Build history of the part. All positions in model axes, mm. Face numbers are marked on the shaded views. A direction names the side the tool comes from. Coordinates: 2 decimals unless noted, no trailing zeros. Order: outer loops, then holes, each group sorted by start corner. A loop starts at its lowest first (then second) coordinate and runs counter-clockwise, first axis right, second up. Notation, with made-up numbers: (-25.75, 57.5) - (-7.75, 57.5) arc R17 ccw to (-7.75, 79.5) - close; hole circle Ø5 at (-19, -26.5). An arc over 180 degrees is marked (long way). One line per item, written item: value.
from build123d import *

# Parameters (mm, degrees)
F0_W           = 15
F0_H           = 2
F1_DEPTH       = 54
F2_W           = 8.5
F2_H           = 15
F3_DEPTH       = 12.5
F5_D           = 3
F5_DEPTH       = 18
F5_CBORE_D     = 6.5
F5_CBORE_DEPTH = 1.5
F5_TIP         = 0.9012909285
F7_D           = 3
F7_DEPTH       = 18
F7_CBORE_D     = 6.5
F7_CBORE_DEPTH = 1.5
F7_TIP         = 0.9012909285
F8_R           = 4
F9_DEPTH       = 10


with BuildPart() as f1:
    # F0 (on Top) → F1 (new body)
    with BuildSketch(Plane.XY):
        with BuildLine():
            Line((0, 5), (0, 0))
            Line((0, 0), (40, 0))
            Line((40, 0), (40, 25))
            Line((40, 25), (0, 25))
            Line((0, 25), (0, 20))
            ThreePointArc((0, 20), (5.3033008589, 17.8033008589), (7.5, 12.5))
            ThreePointArc((7.5, 12.5), (5.3033008589, 7.1966991411), (0, 5))
        make_face()
        Polygon((12.5, 13.5), (12.5, 22), (27.5, 22), (27.5, 13.5), (27.5, 11.5), (27.5, 3), (12.5, 3), (12.5, 11.5), align=None, mode=Mode.SUBTRACT)
        with BuildLine():
            ThreePointArc((0, 25), (-12.5, 12.5), (0, 0))
            Line((0, 0), (0, 5))
            ThreePointArc((0, 5), (-7.5, 12.5), (0, 20))
            Line((0, 20), (0, 25))
        make_face()
        with Locations((20, 12.5)):
            Rectangle(F0_W, F0_H)
    extrude(amount=F1_DEPTH)

    # F2 (on face) → F3 (cut, through all)
    with BuildSketch(Plane.YZ.offset(40)):
        with Locations((7.25, 32.25)):
            Rectangle(F2_W, F2_H)
        with Locations((17.75, 21.75)):
            Rectangle(F2_W, F2_H)
    extrude(amount=-F3_DEPTH, mode=Mode.SUBTRACT)

    # F5
    with Locations(Plane.XZ):
        with Locations((30.5, 32.25)):
            CounterBoreHole(F5_D / 2, F5_CBORE_D / 2, F5_CBORE_DEPTH, depth=F5_DEPTH)
            with Locations((0, 0, -(F5_DEPTH + F5_TIP / 2))):  # 118° drill point
                Cone(0, F5_D / 2, F5_TIP, mode=Mode.SUBTRACT)

    # F7
    with Locations(Plane(origin=(0, 25, 0), x_dir=(-1, 0, 0), z_dir=(0, 1, 0))):
        with Locations((-30.5, 21.75)):
            CounterBoreHole(F7_D / 2, F7_CBORE_D / 2, F7_CBORE_DEPTH, depth=F7_DEPTH)
            with Locations((0, 0, -(F7_DEPTH + F7_TIP / 2))):  # 118° drill point
                Cone(0, F7_D / 2, F7_TIP, mode=Mode.SUBTRACT)

    # F8 (on face) → F9 (cut)
    with BuildSketch(Plane.YZ.offset(40)):
        with Locations((12.5, 47)):
            Circle(F8_R)
        with Locations((12.5, 7)):
            Circle(F8_R)
    extrude(amount=-F9_DEPTH, mode=Mode.SUBTRACT)

    # F11 (on offset) → F12 (revolve)
    with BuildSketch(Plane.XZ.offset(-12.5)):
        Polygon((6.5, 26.6917535926), (7.5, 25.5), (7.5, 28.5), (6.5, 27.3082464074), align=None)
    revolve(axis=Axis((0, 12.5, 27), (0, 0, 1)))


solid = f1.part
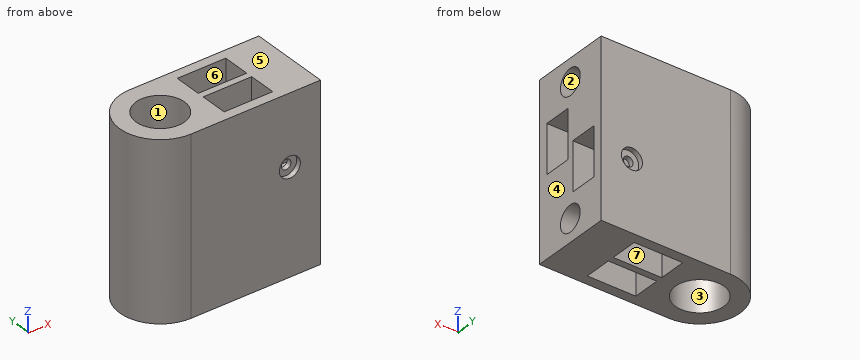
1. Band-saw the part on D-D, the plane z = 10. Give the cut face in (x, y), and give its area (3 significant figures).
Values found:
outline: (0, 0) - (40, 0) - (40, 9.85) - (30, 9.85) - (30, 15.15) - (40, 15.15) - (40, 25) - (0, 25) arc R12.5 ccw to start; hole circle Ø15 at (0, 12.5); hole (12.5, 3) - (27.5, 3) - (27.5, 11.5) - (12.5, 11.5) - close; hole (12.5, 13.5) - (27.5, 13.5) - (27.5, 22) - (12.5, 22) - close
area: 761 mm2
2. Band-saw the part on A-A, the plane y = 12.5. Give the cut face in (x, z).
Values found:
outline: (-12.5, 0) - (-7.5, 0) - (-7.5, 25.5) - (-6.5, 26.69) - (-6.5, 27.31) - (-7.5, 28.5) - (-7.5, 54) - (-12.5, 54) - close; (6.5, 26.69) - (7.5, 25.5) - (7.5, 0) - (40, 0) - (40, 3) - (30, 3) - (30, 11) - (40, 11) - (40, 43) - (30, 43) - (30, 51) - (40, 51) - (40, 54) - (7.5, 54) - (7.5, 28.5) - (6.5, 27.31) - close; hole circle Ø3 at (30.5, 21.75); hole circle Ø3 at (30.5, 32.25)
3. 3-axis set-ups, long thin cutter, end or side, ignore diameter. For the marked faces 1, 2 and 3: which of +Z, -Z, +X, -X, +Y, -Y reach the whole face in a straight line?
Values found:
face 1: +Z
face 2: +X
face 3: -Z
4. Band-saw the part on C-C, the plane x = 14. Give the cut face in (y, z).
Values found:
outline: (0, 0) - (3, 0) - (3, 54) - (0, 54) - close; (11.5, 0) - (13.5, 0) - (13.5, 54) - (11.5, 54) - close; (22, 0) - (25, 0) - (25, 54) - (22, 54) - close
5. Probe line 1 along Y through (x, z) = (15.5, 17.5); line 2 along X through (y, z) = (19.25, 44); line 3 along X through (y, z) = (12.5, 6). List the from-to ranges inside material, lowest first.
Values found:
line 1: y = 0 to 3, 11.5 to 13.5, 22 to 25
line 2: x = -10.52 to -3.27, 3.27 to 12.5, 27.5 to 40
line 3: x = -12.5 to -7.5, 7.5 to 30
6. Band-saw the part on B-B, the plane z = 41.5. Give the cut face in (x, y), and give its area (3 significant figures).
Values found:
outline: (0, 0) - (40, 0) - (40, 25) - (0, 25) arc R12.5 ccw to start; hole circle Ø15 at (0, 12.5); hole (12.5, 3) - (27.5, 3) - (27.5, 11.5) - (12.5, 11.5) - close; hole (12.5, 13.5) - (27.5, 13.5) - (27.5, 22) - (12.5, 22) - close
area: 814 mm2
7. Two-plate mould, pull along X, no slides. Class the marked faces 4, 5, 6 and 7: pulls with the +X half, pulls with the -X half, needs draft (parallel to the pull), parting line crosses it, or undercut.
Values found:
face 4: pulls with the +X half
face 5: needs draft
face 6: undercut
face 7: undercut
8. Flat gauge pins, fed straight in: P1, Ø7, axis at y = 8, z = 9.5, coming from the -X side; P2, Ø2.5, axis at x = 30.5, z = 21.75, coming from the +Y side; P3, Ø12, axis at x = 0, y = 12.5, coming from the -Z side; P4, Ø7, axis at y = 19.5, z = 6.5, coming from the -X side. Where does each tip first touch, or does it go through?
Values found:
P1: stops at x = -12.46
P2: stops at y = 6.85
P3: passes through
P4: stops at x = -12
